Work out the finished part from the listing and answer in its coordinate system (mm). Face numbers are marked on the shaded views. A direction names the side the tool comes from. Coordinates: 2 decimals unless noted, no trailing zeros. Loops run counter-clockwise (first coordinate to the right, second up) from the corner with the lowest first, then second, coordinate; pieces in that order, holes last. Notation, with made-up numbers: (-33, 6) - (2, 6) arc R6 ccw to (2, 13) - close; hole circle Ø7 at (65.5, -8.75). An arc over 180 degrees is marked (long way). Write each question's results on one line, items separated by ' | '. Start each with the question number.
Item 1: Section C-C, the plane x = 4.25 is taken. Write down the section's boundary in (y, z), plus the area to 3 significant figures.
Item 2: Consider probe 1 along X at (y, z) = (1.05, 2.3); probe 2 along Z at (x, y) = (6.75, 0.1); probe 3 along Y at (x, z) = (8.25, 1.3). Determine where each line is inside the solid, lowest interval first. Write a range as [from, to].
Item 3: A tool of negligible diameter and unlimited length cuts with its end or side. For the marked faces 1 and 2, from which of +Z, -Z, +X, -X, +Y, -Y can it reach the whole face along a straight path? Write none if from no direction.
Item 4: Section A-A, the plane z = 0 is taken. Write down the section's boundary in (x, y) (3 decimals), plus the area to 3 significant figures.
Item 5: Each of these flat-tipped pins is pushed along its axis until it touches: pin 1 Ø1 at (x, z) = (8, 0) entering from -Y; pin 2 Ø1 at (x, y) = (7, -1) entering from -Z; pin 3 Ø0.9 at (x, y) = (0.5, -1) entering from -Z. Where does it stop, or does it pass through?
from build123d import *

# Parameters (mm, degrees)
CROSSRECESS_DEPTH = 0.825
DRAFT9_ANGLE      = 30
FILLET5_R         = 0.3


with BuildPart() as part:
    # Sketch1 → Base (revolve)
    with BuildSketch(Plane.XY):
        Polygon((10, 1.5), (2.65, 1.5), (1.65, 1.5), (0.55, 2.6), (0, 2.6), (0, 0), (10, 0), align=None)
    revolve(axis=Axis((4.515812911, 0, 0), (-1, 0, 0)))

    # Sketch6 → CrossRecess (cut)
    with BuildSketch(Plane(origin=(0, 0, 0), x_dir=(0, 0, -1), z_dir=(1, 0, 0))):
        Polygon((0.32, 0.32), (0.32, 1.6), (-0.32, 1.6), (-0.32, 0.32), (-1.6, 0.32), (-1.6, -0.32), (-0.32, -0.32), (-0.32, -1.6), (0.32, -1.6), (0.32, -0.32), (1.6, -0.32), (1.6, 0.32), align=None)
    extrude(amount=CROSSRECESS_DEPTH, mode=Mode.SUBTRACT)

    # Draft9
    draft9_faces = [part.faces().sort_by_distance(p)[0] for p in [
        (0.4125, 1.6, 0),
        (0.4125, 0, 1.6),
        (0.4125, -1.6, 0),
        (0.4125, 0, -1.6),
    ]]
    draft(draft9_faces, Plane(origin=(0, 2.6, 0), x_dir=(0, 0, -1), z_dir=(-1, 0, 0)), DRAFT9_ANGLE)

    # Fillet5
    fillet5_edges = [part.edges().sort_by_distance(p)[0] for p in [
        (0.4125, 0.32, 0.32),
        (0.4125, -0.32, 0.32),
        (0.4125, -0.32, -0.32),
        (0.4125, 0.32, -0.32),
    ]]
    fillet(fillet5_edges, radius=FILLET5_R)


solid = part.part
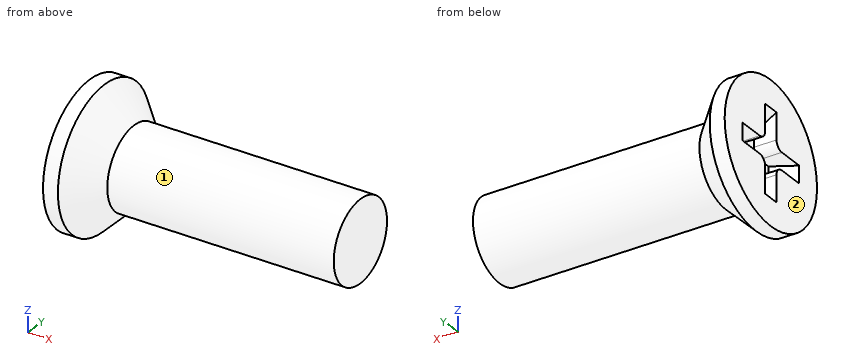
Answer key:
1) outline: circle Ø3 at (0, 0) | area: 7.07 mm^2
2) probe 1: x = [0, 0.62] | probe 2: z = [-1.5, 1.5] | probe 3: y = [-0.75, 0.75]
3) face 1: +X | face 2: +Z, -Z, -X, +Y, -Y
4) outline: (0, -2.6) - (0.55, -2.6) - (1.65, -1.5) - (10, -1.5) - (10, 1.5) - (1.65, 1.5) - (0.55, 2.6) - (0, 2.6) - (0, 1.6) - (0.825, 1.124) - (0.825, -1.124) - (0, -1.6) - close | area: 30.2 mm^2
5) pin 1: stops at y = -1.5 | pin 2: stops at z = -1.41 | pin 3: stops at z = -2.54
